Check sheet for the modelled part. Datum: model origin and axes. Units: mm. Face numbers are marked on the shaded views. A direction names the side the tool comes from. Coordinates: 2 decimals unless noted, no trailing zeros. Write each loop counter-clockwise with the first axis right and the second up, starting at its lowest first coordinate (ties: lowest second). Pieces come first, ordered by that corner, then holes. Notation, with made-up numbers: (7, 26.5) -> (47, 26.5) arc R25 cw to (47, 48.5) -> close; hole circle Ø1 at (20.25, 51). An arc over 180 degrees is marked (long way). One line per item, written item: value. Start each with the question number.
1) Sectioned sample at A-A on y = 40.5. Enter the section's corners in (x, z), plus the area to 3 significant figures.
2) Sectioned sample at C-C on z = 0. Enter the section's corners in (x, y).
3) Draft check along Z on the marked faces 1, 2 and 3. Enter one of: +Z half, -Z half, draft (parallel to the pull), parting line (faces both ways), or undercut.
4) Gauge pin test, flat ends, axial feed: P1, Ø3, axis at y = 17.5, z = 11, coming from the +X side; P2, Ø5, axis at y = 22.5, z = -21.5, coming from the +X side; P3, Ø3, axis at y = 25.5, z = -14.5, coming from the -X side. Record the tip position at first contact, or that the pin passes through.
5) Sectioned sample at B-B on x = 0. Enter the section's corners in (y, z).
6) Scan lines: line 1 along X through (y, z) = (10, 0); line 2 along Z through (x, y) = (0, 14); line 3 along Y through (x, z) = (-15.5, 25.5). Record each from-to range of solid material in increasing order. Write a range as [from, to].
7) Set-up check for the marked faces 4, 5 and 6: record each of +Z, -Z, +X, -X, +Y, -Y from which the full face is reachable in a straight line by a thin tool's end or side.
8) Sectioned sample at D-D on y = 32. Enter the section's corners in (x, z).
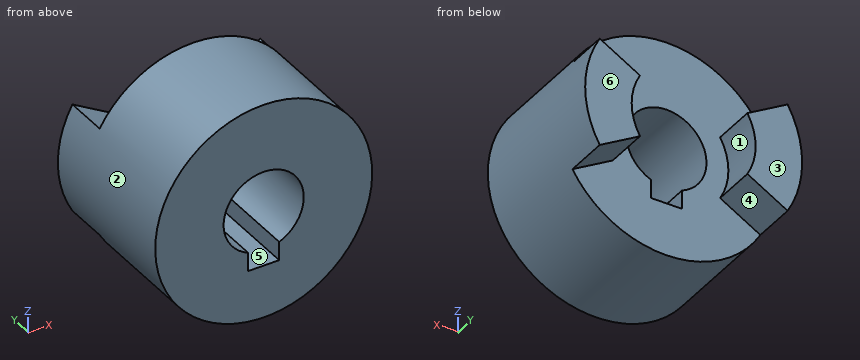
```python
from build123d import *

# Parameters (mm, degrees)
SKETCH1_R           = 35
BOSS_EXTRUDE1_DEPTH = 50
CUT_EXTRUDE1_START  = -14
CUT_EXTRUDE1_DEPTH  = 14
CUT_EXTRUDE2_DEPTH  = 71.356236397
CUT_EXTRUDE8_START  = 36
SKETCH10_R          = 20
CUT_EXTRUDE8_DEPTH  = 35.356236397


with BuildPart() as part:
    # Sketch1 → Boss-Extrude1 (new body)
    with BuildSketch(Plane(origin=(0, 0, 0), x_dir=(1, 0, 0), z_dir=(0, 1, 0))):
        with Locations(Location((0, 0, 0), (0, 0, 270))):
            Circle(SKETCH1_R)
    extrude(amount=BOSS_EXTRUDE1_DEPTH)

    # Sketch2 → Cut-Extrude1 (cut)
    with BuildSketch(Plane(origin=(0, 50, 0), x_dir=(1, 0, 0), z_dir=(0, 1, 0)).offset(CUT_EXTRUDE1_START)):
        with BuildLine():
            Line((-10.392304845, -6), (-30.310889132, -17.5))
            ThreePointArc((-30.310889132, -17.5), (0, -35), (30.310889132, -17.5))
            Line((30.310889132, -17.5), (10.392304845, -6))
            ThreePointArc((10.392304845, -6), (0, -12), (-10.392304845, -6))
        make_face()
    cut_extrude1 = extrude(amount=CUT_EXTRUDE1_DEPTH, mode=Mode.SUBTRACT)

    # Mirror2: Cut-Extrude1 across plane
    add(cut_extrude1.mirror(Plane.XY), mode=Mode.SUBTRACT)

    # Sketch3 → Cut-Extrude2 (cut, through all)
    with BuildSketch(Plane(origin=(0, 0, 0), x_dir=(1, 0, 0), z_dir=(0, 1, 0))):
        with BuildLine():
            Line((5, 11.924130996), (5, 17.93))
            Line((5, 17.93), (-5, 17.93))
            Line((-5, 17.93), (-5, 11.924130996))
            ThreePointArc((-5, 11.924130996), (0, -12.93), (5, 11.924130996))
        make_face()
    extrude(amount=CUT_EXTRUDE2_DEPTH, mode=Mode.SUBTRACT)

    # Sketch10 → Cut-Extrude8 (cut, through all)
    with BuildSketch(Plane(origin=(0, 0, 0), x_dir=(1, 0, 0), z_dir=(0, 1, 0)).offset(CUT_EXTRUDE8_START)):
        Circle(SKETCH10_R)
    extrude(amount=CUT_EXTRUDE8_DEPTH, mode=Mode.SUBTRACT)


solid = part.part
```
Answers:
1. outline: (-30.31, -17.5) -> (-17.32, -10) arc R20 cw to (-17.32, 10) -> (-30.31, 17.5) arc R35 ccw to start; (17.32, -10) -> (30.31, -17.5) arc R35 ccw to (30.31, 17.5) -> (17.32, 10) arc R20 cw to start
1. area: 864 mm2
2. outline: (-35, 0) -> (-12.93, 0) -> (-12.93, 36) -> (-20, 36) -> (-20, 50) -> (-35, 50) -> close; (12.93, 0) -> (35, 0) -> (35, 50) -> (20, 50) -> (20, 36) -> (12.93, 36) -> close
3. face 1: undercut
3. face 2: parting line
3. face 3: draft
4. P1: stops at x = 33.69
4. P2: stops at x = 29.39
4. P3: stops at x = -32.5
5. outline: (0, -35) -> (36, -35) -> (36, -17.93) -> (0, -17.93) -> close; (0, 12.93) -> (36, 12.93) -> (36, 35) -> (0, 35) -> close
6. line 1: x = [-35, -12.93], [12.93, 35]
6. line 2: z = [-35, -17.93], [12.93, 35]
6. line 3: y = [0, 36]
7. face 4: -Z, +Y
7. face 5: +Y, -Y
7. face 6: +Z, -Z, +X, -X, +Y
8. outline: circle Ø70 at (0, 0); hole (-5, -17.93) -> (5, -17.93) -> (5, -11.92) arc R12.93 ccw (long way) to (-5, -11.92) -> close
